Build history of the part. All positions in model axes, mm. Give positions to 0.01 mm unless a question says otherwise; leave off trailing zeros. Write each loop counter-clockwise with the first axis right and the second up, starting at its lowest first coordinate (ties: lowest second). Pieces come first, ordered by that corner, then holes. Notation, with made-up numbers: M 76.25,-18 L 111.25,-18 A31 cw 111.25,6 Z; hole C 35.5,-15.75 d7. An arc over 180 degrees is marked long. Return JSON: item names as keys, results as strings. Group by question number.
Q1. Wall check: probe 1 along X at (y, z) = (3.25, 100); probe 2 along Z at (x, y) = (162.5, 4.5); probe 3 along X at (y, z) = (-1.5, 14). Give the ranges that are in metal, low to high.
Q2. Band-saw the part on D-D, the plane z = 100. Give the cut face in (x, y), then the cut area to 3 significant figures.
Q3. Band-saw the part on A-A, the plane x = -162.5. Give the cut face in (y, z), then the cut area to 3 significant figures.
Q4. Band-saw the part on C-C, the plane y = 2.75. Count the separate pieces of the cut face and the enclosed holes in it, then the cut area to 3 significant figures.
Q5. Band-saw the part on B-B, the plane z = -12. Give the cut face in (x, y).
from build123d import *

# Parameters (mm, degrees)
SKETCH1_W               = 350
SKETCH1_H               = 220
BOSS_EXTRUDE1_DEPTH     = 7.5
SKETCH2_R               = 3.5
CUT_EXTRUDE1_DEPTH      = 208.243817761
MIRROR2_COPY_1_SKETCH_R = 3.5
MIRROR2_COPY_1_DEPTH    = 208.243817761
CUT_EXTRUDE2_DEPTH      = 208.243817761
SKETCH4_R               = 3.5
CUT_EXTRUDE5_DEPTH      = 208.243817761
MIRROR4_COPY_1_SKETCH_R = 3.5
MIRROR4_COPY_1_DEPTH    = 208.243817761


with BuildPart() as part:
    # Sketch1 → Boss-Extrude1 (new, symmetric)
    with BuildSketch(Plane(origin=(0, 0, 0), x_dir=(1, 0, 0), z_dir=(0, 1, 0))):
        Rectangle(SKETCH1_W, SKETCH1_H)
    extrude(amount=BOSS_EXTRUDE1_DEPTH, both=True)

    # Sketch2 → Cut-Extrude1 (cut, symmetric)
    with BuildSketch(Plane(origin=(0, 7.5, 0), x_dir=(1, 0, 0), z_dir=(0, 1, 0))):
        with Locations(Location((-100, 100, 0), (0, 0, 270))):
            Circle(SKETCH2_R)
    cut_extrude1 = extrude(amount=CUT_EXTRUDE1_DEPTH, both=True, mode=Mode.SUBTRACT)

    # Mirror1: Cut-Extrude1 across plane
    add(cut_extrude1.mirror(Plane.XY), mode=Mode.SUBTRACT)

    # Mirror2: Cut-Extrude1 across plane
    add(cut_extrude1.mirror(Plane(origin=(0, 0, 0), x_dir=(0, 0, 1), z_dir=(1, 0, 0))), mode=Mode.SUBTRACT)

    # Mirror2 copy 1 sketch → Mirror2 copy 1 (cut, symmetric)
    with BuildSketch(Plane(origin=(0, 7.5, 0), x_dir=(-1, 0, 0), z_dir=(0, 1, 0))):
        with Locations(Location((-100, 100, 0), (0, 0, 270))):
            Circle(MIRROR2_COPY_1_SKETCH_R)
    extrude(amount=MIRROR2_COPY_1_DEPTH, both=True, mode=Mode.SUBTRACT)

    # Sketch3 → Cut-Extrude2 (cut, symmetric)
    with BuildSketch(Plane(origin=(0, 7.5, 0), x_dir=(1, 0, 0), z_dir=(0, 1, 0))):
        with BuildLine():
            Line((-167.5, -25), (-167.5, 25))
            ThreePointArc((-167.5, 25), (-162.5, 30), (-157.5, 25))
            Line((-157.5, 25), (-157.5, -25))
            ThreePointArc((-157.5, -25), (-162.5, -30), (-167.5, -25))
        make_face()
    cut_extrude2 = extrude(amount=CUT_EXTRUDE2_DEPTH, both=True, mode=Mode.SUBTRACT)

    # Sketch4 → Cut-Extrude5 (cut, symmetric)
    with BuildSketch(Plane(origin=(0, 7.5, 0), x_dir=(1, 0, 0), z_dir=(0, 1, 0))):
        with Locations(Location((-162.5, 100, 0), (0, 0, 270))):
            Circle(SKETCH4_R)
    cut_extrude5 = extrude(amount=CUT_EXTRUDE5_DEPTH, both=True, mode=Mode.SUBTRACT)

    # Mirror3: Cut-Extrude5 across plane
    add(cut_extrude5.mirror(Plane.XY), mode=Mode.SUBTRACT)

    # Mirror4: Cut-Extrude5 across plane
    add(cut_extrude5.mirror(Plane(origin=(0, 0, 0), x_dir=(0, 0, 1), z_dir=(1, 0, 0))), mode=Mode.SUBTRACT)

    # Mirror4 copy 1 sketch → Mirror4 copy 1 (cut, symmetric)
    with BuildSketch(Plane(origin=(0, 7.5, 0), x_dir=(-1, 0, 0), z_dir=(0, 1, 0))):
        with Locations(Location((-162.5, 100, 0), (0, 0, 270))):
            Circle(MIRROR4_COPY_1_SKETCH_R)
    extrude(amount=MIRROR4_COPY_1_DEPTH, both=True, mode=Mode.SUBTRACT)

    # Mirror5: Cut-Extrude2 across plane
    add(cut_extrude2.mirror(Plane(origin=(0, 0, 0), x_dir=(0, 0, 1), z_dir=(1, 0, 0))), mode=Mode.SUBTRACT)


solid = part.part
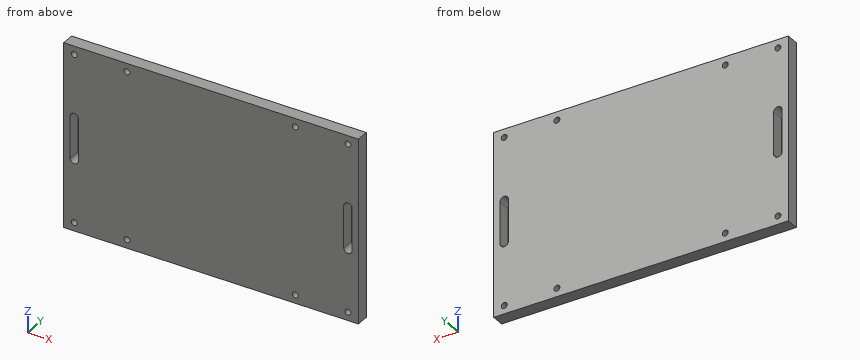
From the geometry:
{
 "1": {"probe 1": "x = -175 to -166, -159 to -103.5, -96.5 to 96.5, 103.5 to 159, 166 to 175", "probe 2": "z = -110 to -103.5, -96.5 to -30, 30 to 96.5, 103.5 to 110", "probe 3": "x = -175 to -167.5, -157.5 to 157.5, 167.5 to 175"},
 "2": {"outline": "M -175,-7.5 L -166,-7.5 L -166,7.5 L -175,7.5 Z; M -159,-7.5 L -103.5,-7.5 L -103.5,7.5 L -159,7.5 Z; M -96.5,-7.5 L 96.5,-7.5 L 96.5,7.5 L -96.5,7.5 Z; M 103.5,-7.5 L 159,-7.5 L 159,7.5 L 103.5,7.5 Z; M 166,-7.5 L 175,-7.5 L 175,7.5 L 166,7.5 Z", "area": "4,830 mm^2"},
 "3": {"outline": "M -7.5,-110 L 7.5,-110 L 7.5,-103.5 L -7.5,-103.5 Z; M -7.5,-96.5 L 7.5,-96.5 L 7.5,-30 L -7.5,-30 Z; M -7.5,30 L 7.5,30 L 7.5,96.5 L -7.5,96.5 Z; M -7.5,103.5 L 7.5,103.5 L 7.5,110 L -7.5,110 Z", "area": "2,190 mm^2"},
 "4": {"separate pieces": "1", "enclosed holes": "10", "area": "75,500 mm^2"},
 "5": {"outline": "M -175,-7.5 L -167.5,-7.5 L -167.5,7.5 L -175,7.5 Z; M -157.5,-7.5 L 157.5,-7.5 L 157.5,7.5 L -157.5,7.5 Z; M 167.5,-7.5 L 175,-7.5 L 175,7.5 L 167.5,7.5 Z"}
}
